Geometry: final body of the model. Coordinates: model frame, mm. Face numbers are marked on the shaded views. A direction names the side the tool comes from. Give positions to 0.01 mm unless a question says otherwise; leave off trailing zeros. Write each loop counter-clockwise with the first axis right and the second up, starting at its lowest first coordinate (ties: lowest second). Pieces come first, ordered by that corner, then holes.
Q1. Draft query along Y for the marked faces 1, 2 and 3. Return one class per face: pulls with the +Y half, pulls with the -Y half, needs draft (parallel to the pull), parting line crosses it, or undercut.
Q2. Cut plane B-B on y = 16.75. Return the cut outline in (x, z).
Q3. Cut plane C-C on y = 7.75. Return the cut outline in (x, z).
Q4. Line query: L1, parallel to Z at x = 0, y = 13.15; L2, parallel to X at y = 5, z = 0. Output: solid intervals per line, ascending.
Q5. Pin query (flat end, axial travel): pin 1 (1.2 mm diameter, centred on x = 8, z = 0, fed in from -Y); pin 2 (3 mm diameter, centred on x = 0, z = 0, fed in from +Y); pin 3 (2.5 mm diameter, centred on x = 6.93, z = 4, fed in from +Y); pin 4 (5 mm diameter, centred on x = -9.5, y = 10, fed in from +Z). Return the tip coordinate at first contact, or that it passes through.
Q6. Reachability of the marked faces 4 and 5 from +Z, -Z, +X, -X, +Y, -Y: full face, straight path, thin tool, end or side. Return the list, or none.
Autodesk Inventor part; units mm, degrees
ref_plane "YZ Plane" through (0, 0, 0) normal (1, 0, 0) x (0, 1, 0)
ref_plane "XZ Plane" through (0, 0, 0) normal (0, 1, 0) x (-1, 0, 0)
ref_plane "XY Plane" through (0, 0, 0) normal (0, 0, 1) x (1, 0, 0)
sketch "Sketch1" plane through (0, 0, 0) normal (0, 1, 0) x (-1, 0, 0)
  circle A0 centre (0, 0) radius 30
  circle A1 centre (0, 0) radius 2.5
  dimension "d0" = 60
  dimension "d1" = 5
extrude "Extrusion1" add sketch "Sketch1" along normal blind 2
sketch "Sketch2" plane through (0, 2, 0) normal (0, 1, 0) x (1, 0, 0)
  circle A0 centre (0, 0) radius 2.5
  circle A1 centre (0, 0) radius 6.5
  dimension "d4" = 13
extrude "Extrusion2" add sketch "Sketch2" along normal blind 10
sketch "Sketch3" plane through (0, 12, 0) normal (0, 1, 0) x (1, 0, 0)
  circle A0 centre (0, 0) radius 30
  circle A1 centre (0, 0) radius 2.5
extrude "Extrusion3" add sketch "Sketch3" along normal blind 2
sketch "Sketch4" plane through (0, 0, 0) normal (1, 0, 0) x (0, 1, 0)
  line L0 (2, 6.5) -> (12, 6.5)
  line L1 (2, 6.5) -> (3.5, 6.5)
  line L2 (2, -30) -> (2, 30)
  line L3 (3.5, 6.5) -> (2, 30)
  line L4 (12, 6.5) -> (10.5, 6.5)
  line L5 (12, -30) -> (12, 30)
  line L6 (10.5, 6.5) -> (12, 30)
  line L7 (-2.8, 0) -> (16.8, 0)
  point P0 (0, 0)
  dimension "d9" = 1.5
  dimension "d10" = 1.5
revolve "Revolution1" add sketch "Sketch4" angle 360 about axis through (0, -10, 0) along (0, 1, 0) contours L2 L3 L0 | L6 L5 L0
sketch "Sketch6" plane through (0, 0, 0) normal (1, 0, 0) x (0, 1, 0)
  line L0 (0, -30) -> (0, 30)
  line L1 (0, 30) -> (1, 30)
  line L2 (0, 30) -> (2, 30)
  line L3 (1, 30) -> (2.1063, 28.3339)
  line L4 (2, 30) -> (3.5, 6.5)
  line L5 (2.1063, 28.3339) -> (1, 28.3339)
  line L6 (1, 28.3339) -> (1, 30)
  line L7 (14, -30) -> (14, 30)
  line L8 (14, 30) -> (13, 30)
  line L9 (12, 30) -> (14, 30)
  line L10 (13, 30) -> (11.8937, 28.3339)
  line L11 (10.5, 6.5) -> (12, 30)
  line L12 (11.8937, 28.3339) -> (14, 28.3339)
  line L13 (14, 28.3339) -> (14, 30)
  line L14 (13, 30) -> (13, 28.3339)
  line L15 (-2.8, 0) -> (16.8, 0)
  point P0 (0, 0)
  dimension "d12" = 1
  dimension "d13" = 2
revolve "Revolution2" cut sketch "Sketch6" angle 360 about axis through (0, -10, 0) along (0, 1, 0) contours L2 L4 L3 | L10 L11 L9
sketch "Sketch7" plane through (0, 14, 0) normal (0, 1, 0) x (1, 0, 0)
  circle A0 centre (0, 0) radius 2.5
  circle A1 centre (0, 0) radius 5
  dimension "d15" = 10
extrude "Extrusion4" add sketch "Sketch7" along normal blind 10
ref_plane "Work Plane1" through (0, 7, 0) normal (0, 1, 0) x (1, 0, 0)
sketch "Sketch8" plane through (0, 0, 0) normal (0, -1, 0) x (1, 0, 0)
  line L0 (0, 0) -> (8, 0)
  circle A0 centre (8, 0) radius 1
  circle A1 centre (6.9282, 4) radius 1
  dimension "d18" = 8
  dimension "d21" = 30
  dimension "d25" = 2
extrude "Extrusion5" cut sketch "Sketch8" against normal up to surface
properties part number "spool"
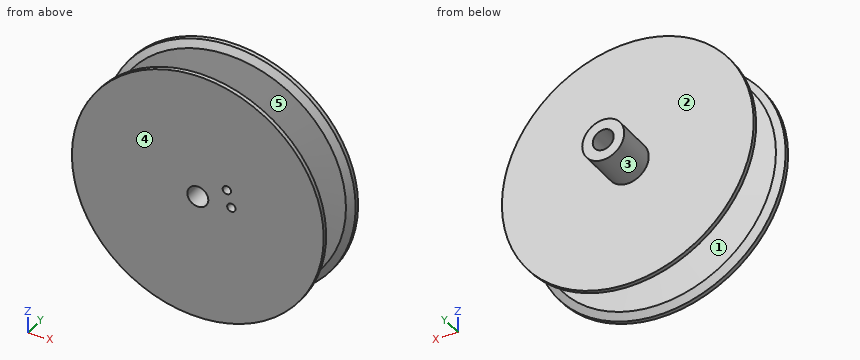
Data:
1. face 1: undercut
1. face 2: pulls with the +Y half
1. face 3: needs draft
2. outline: circle Ø10 at (0, 0); hole circle Ø5 at (0, 0)
3. outline: circle Ø13 at (0, 0); hole circle Ø5 at (0, 0)
4. L1: z = -30 to -2.5, 2.5 to 30
4. L2: x = -6.5 to -2.5, 2.5 to 6.5
5. pin 1: stops at y = 10.56
5. pin 2: passes through
5. pin 3: stops at y = 14
5. pin 4: stops at z = 27.75
6. face 4: +Z, -Z, +X, -X, -Y
6. face 5: none
